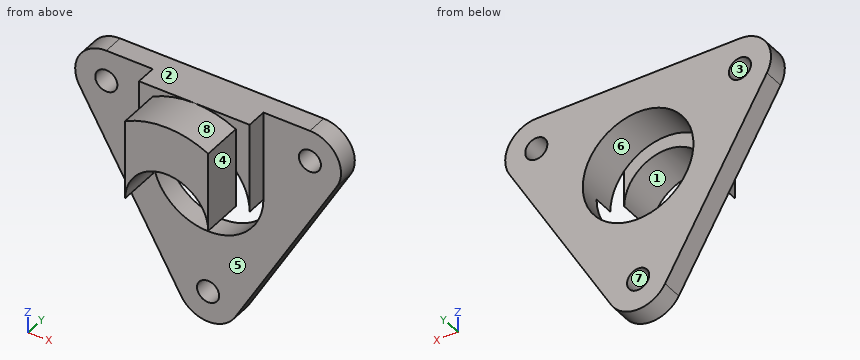
```python
from build123d import *

# Parameters (mm, degrees)
EXTRUDE_1_DEPTH   = 6
EXTRUDE_2_DEPTH   = 3
SKETCH_4_R        = 8
EXTRUDE_3_DEPTH   = 3
OTHER_START       = -10.160108376
OTHER_1_OUTLINE_R = 1.6
OTHER_1_DEPTH     = 3


# Read off the part's stored shape, not the designer's step: 高级异型孔1
with BuildPart() as part:
    # 草图1 → 凸台-拉伸1 (new body)
    with BuildSketch(Plane(origin=(0, -13.160108376, 0), x_dir=(1, 0, 0), z_dir=(0, 1, 0))):
        with BuildLine():
            Line((-6, 0), (-6, -11.532562595))
            ThreePointArc((-6, -11.532562595), (0, -13), (6, -11.532562595))
            Line((6, -11.532562595), (6, 0))
            ThreePointArc((6, 0), (0, -6), (-6, 0))
        make_face()
    extrude(amount=-EXTRUDE_1_DEPTH)

    # 草图2 → 凸台-拉伸2 (add)
    with BuildSketch(Plane(origin=(0, -13.160108376, 0), x_dir=(1, 0, 0), z_dir=(0, 1, 0))):
        with BuildLine():
            Line((-8, 0), (-8, -13))
            Line((-8, -13), (8, -13))
            Line((8, -13), (8, 0))
            ThreePointArc((8, 0), (0, -8), (-8, 0))
        make_face()
    extrude(amount=EXTRUDE_2_DEPTH)

    # 草图4 → 凸台-拉伸3 (add)
    with BuildSketch(Plane(origin=(0, -10.160108376, -27), x_dir=(1, 0, 0), z_dir=(0, 1, 0))):
        with BuildLine():
            Line((-3.897114317, -7.75), (-18.619546181, -33.25))
            ThreePointArc((-18.619546181, -33.25), (-18.619546181, -37.75), (-14.722431864, -40))
            Line((-14.722431864, -40), (14.722431864, -40))
            ThreePointArc((14.722431864, -40), (18.619546181, -37.75), (18.619546181, -33.25))
            Line((18.619546181, -33.25), (3.897114317, -7.75))
            ThreePointArc((3.897114317, -7.75), (0, -5.5), (-3.897114317, -7.75))
        make_face()
        with Locations((0, -27)):
            Circle(SKETCH_4_R, mode=Mode.SUBTRACT)
    extrude(amount=EXTRUDE_3_DEPTH)

    # 高级异型孔1 outline → 高级异型孔1 (cut)
    with BuildSketch(Plane(origin=(0, 0, 0), x_dir=(1, 0, 0), z_dir=(0, 1, 0)).offset(OTHER_START)):
        with Locations((-14.722431864, -8.5)):
            Circle(OTHER_1_OUTLINE_R)
        with Locations((14.722431864, -8.5)):
            Circle(OTHER_1_OUTLINE_R)
        with Locations((0, 17)):
            Circle(OTHER_1_OUTLINE_R)
    extrude(amount=OTHER_1_DEPTH, mode=Mode.SUBTRACT)


solid = part.part
```
Here's how the part is built. I have some questions about the finished solid (model axes, mm). Face numbers are marked on the shaded views. A direction names the side the tool comes from. Coordinates: 2 decimals unless noted, no trailing zeros. Order: outer loops, then holes, each group sorted by start corner. A loop starts at its lowest first (then second) coordinate and runs counter-clockwise, first axis right, second up. Notation, with made-up numbers: (11, 29.5) -> (41, 29.5) arc R25 cw to (41, 45.5) -> close; hole circle Ø4 at (-35.75, 4). An arc over 180 degrees is marked (long way). Return JSON: item names as keys, results as strings.
1) I'm going to push flat-ended pins straight in: P1, Ø3.5, axis at y = -11, z = 6, coming from the +X side; P2, Ø2.5, axis at y = -11.5, z = 4, coming from the -X side; P3, Ø4, axis at x = -14.72, z = 8.5, coming from the +Y side; P4, Ø2, axis at y = -13, z = -10, coming from the -X side. Where does each tip first touch, or does it pass through?
Conclusion:
{"P1": "stops at x = 19.12", "P2": "stops at x = -8", "P3": "stops at y = -7.16", "P4": "passes through"}
2) If we section it at A-A on y = -8.75: List the corners of the cut face in (x, z) for me.
Conclusion:
{"outline": "(-18.62, 6.25) -> (-3.9, -19.25) arc R4.5 ccw to (3.9, -19.25) -> (18.62, 6.25) arc R4.5 ccw to (14.72, 13) -> (-14.72, 13) arc R4.5 ccw to start; hole circle Ø3.2 at (-14.72, 8.5); hole circle Ø16 at (0, 0); hole circle Ø3.2 at (0, -17); hole circle Ø3.2 at (14.72, 8.5)"}
3) If we section it at D-D on z = -17: List the corners of the cut face in (x, y) for me.
Conclusion:
{"outline": "(-5.2, -10.16) -> (-1.6, -10.16) -> (-1.6, -7.16) -> (-5.2, -7.16) -> close; (1.6, -10.16) -> (5.2, -10.16) -> (5.2, -7.16) -> (1.6, -7.16) -> close"}
4) Thinking about a two-plate mould opening in Z: for the marked faces 1, 2, 3 and 4, which applies, +Z half, -Z half, draft (parallel to the pull), parting line (faces both ways), or undercut?
Conclusion:
{"face 1": "-Z half", "face 2": "+Z half", "face 3": "undercut", "face 4": "draft"}
5) If we section it at B-B on z = 8.5: List the corners of the cut face in (x, y) for me, plus the area to 3 significant figures.
Conclusion:
{"outline": "(-19.22, -10.16) -> (-16.32, -10.16) -> (-16.32, -7.16) -> (-19.22, -7.16) -> close; (-13.12, -10.16) -> (-8, -10.16) -> (-8, -13.16) -> (-6, -13.16) -> (-6, -19.16) -> (6, -19.16) -> (6, -13.16) -> (8, -13.16) -> (8, -10.16) -> (13.12, -10.16) -> (13.12, -7.16) -> (-13.12, -7.16) -> close; (16.32, -10.16) -> (19.22, -10.16) -> (19.22, -7.16) -> (16.32, -7.16) -> close", "area": "216 mm²"}
6) On a 3-axis mill with a long thin cutter (end or side, diameter ignored), from which of +Z, -Z, +X, -X, +Y, -Y can I reach the whole of each face in a straight line? I mean the marked faces 5, 6, 7 and 8. Say none if no direction works.
Conclusion:
{"face 5": "-Z, -Y", "face 6": "+Y", "face 7": "+Y, -Y", "face 8": "+Z, -Y"}
7) If I drill on probe 1 along X at (y, z) = (-8.4, 8.5); probe 2 along X at (y, z) = (-9.75, -5.5); probe 3 along X at (y, z) = (-16, 9), over which ranges is the centre line in solid material (lowest first)?
Conclusion:
{"probe 1": "x = -19.22 to -16.32, -13.12 to 13.12, 16.32 to 19.22", "probe 2": "x = -11.84 to -5.81, 5.81 to 11.84", "probe 3": "x = -6 to 6"}
8) If we section it at C-C on z = 4.5: List the corners of the cut face in (x, y) for me, plus the area to 3 significant figures.
Conclusion:
{"outline": "(-17.61, -10.16) -> (-8, -10.16) -> (-8, -13.16) -> (-6.61, -13.16) -> (-6.61, -7.16) -> (-17.61, -7.16) -> close; (-6, -19.16) -> (-3.97, -19.16) -> (-3.97, -13.16) -> (-6, -13.16) -> close; (3.97, -19.16) -> (6, -19.16) -> (6, -13.16) -> (3.97, -13.16) -> close; (6.61, -13.16) -> (8, -13.16) -> (8, -10.16) -> (17.61, -10.16) -> (17.61, -7.16) -> (6.61, -7.16) -> close", "area": "98.7 mm²"}
